from build123d import *

# Parameters (mm, degrees)
F0_W     = 1000
F0_H     = 100
F1_DEPTH = 50
F3_R     = 5
F4_DEPTH = 25
F2_R     = 5
F5_DEPTH = 50
F6_R     = 5
F7_DEPTH = 50
F8_R     = 49.99999


# Not quite as in the source:
# - a fillet or chamfer is up to 0.001 mm smaller than in the source, because OpenCascade refuses the exact size


with BuildPart() as f1:
    # F0 (on Front) → F1 (new body)
    with BuildSketch(Plane.XZ):
        Rectangle(F0_W, F0_H)
    extrude(amount=F1_DEPTH)

    # F3 (on face) → F4 (cut)
    with BuildSketch(Plane.XY.offset(50)):
        with Locations((-100, -25)):
            Circle(F3_R)
        with Locations((-50, -25)):
            Circle(F3_R)
    extrude(amount=-F4_DEPTH, mode=Mode.SUBTRACT)

    # F2 (on face) → F5 (cut)
    with BuildSketch(Plane.XZ.offset(50)):
        with Locations((-50, 0)):
            Circle(F2_R)
        Circle(F2_R)
        with Locations((-350, 0)):
            Circle(F2_R)
        with Locations((-300, 0)):
            Circle(F2_R)
    extrude(amount=-F5_DEPTH, mode=Mode.SUBTRACT)

    # F6 (on face) → F7 (cut)
    with BuildSketch(Plane(origin=(0, 0, 0), x_dir=(-1, 0, 0), z_dir=(0, 1, 0))):
        with Locations((-225, -25)):
            Circle(F6_R)
        with Locations((-175, -25)):
            Circle(F6_R)
        with Locations((-225, 25)):
            Circle(F6_R)
        with Locations((-175, 25)):
            Circle(F6_R)
    extrude(amount=-F7_DEPTH, mode=Mode.SUBTRACT)

    # F8 (radius 50 in the source; OpenCascade refuses exactly that, so slightly less here)
    f8_edges = [f1.edges().sort_by_distance(p)[0] for p in [
        (-500, -25, 50),
        (-500, -25, -50),
    ]]
    fillet(f8_edges, radius=F8_R)


solid = f1.part
Work out the finished part from the listing and answer in its coordinate system (mm). Coordinates: 2 decimals unless noted, no trailing zeros. Use one line per item in the form item = value. Start each with the question number.
1. The part is cut by section A-A (y = -10). Give the number of separate pieces and of enclosed holes in the cut face, plus the area to 3 significant figures.
2. Each of these flat-tipped pins is pushed along its axis until it touches: P1, Ø11.5, axis at x = -300, z = 0, coming from the +Y side; P2, Ø4, axis at y = -25.5, z = -11.5, coming from the -X side; P3, Ø6, axis at x = -100, y = -25, coming from the +Z side. Where does it stop, or does it pass through?
3. Straight lines are drawn through the part: probe 1 along Z at (x, y) = (225, -25); probe 2 along Z at (x, y) = (0, -13); probe 3 along Y at (x, z) = (-50, 34). For each, find the intervals that lie inside material, in ascending order. Write a range as from..to.
Evaluation:
q1.separate_pieces = 1
q1.enclosed_holes = 8
q1.area = 98,300 mm^2
q2.P1 = 0
q2.P2 = -499.09
q2.P3 = 25
q3.probe_1 = -50..-30, -20..20, 30..50
q3.probe_2 = -50..-5, 5..50
q3.probe_3 = -50..-30, -20..0
